Can you work these out from the model? Positions are in its coordinate system, mm. A direction names the side the tool comes from. Round coordinates to 2 decimals unless told otherwise and drop trailing zeros. Loops run counter-clockwise (first coordinate to the right, second up) from the corner with the lowest first, then second, coordinate; pieces in that order, holes last. Notation, with made-up numbers: (49, 35.25) - (103, 35.25) arc R33 ccw to (103, 70.25) - close; hole circle Ø5 at (75, -37.5). An arc over 180 degrees is marked (long way). Answer as CSV lines item,"result".
```python
from build123d import *

# Parameters (mm, degrees)
F0_W     = 127
F0_H     = 76.2
F1_DEPTH = 12
F2_R     = 5
F3_SIZE  = 2
F4_T     = -1


with BuildPart() as f1:
    # F0 (on Top) → F1 (new body)
    with BuildSketch(Plane.XY):
        with Locations((-63.5, -38.1)):
            Rectangle(F0_W, F0_H)
    extrude(amount=F1_DEPTH)

    # F2
    f2_edges = [f1.edges().sort_by_distance(p)[0] for p in [
        (-63.5, -76.2, 0),
    ]]
    fillet(f2_edges, radius=F2_R)

    # F3
    f3_edges = [f1.edges().sort_by_distance(p)[0] for p in [
        (0, -76.2, 8.5),
        (-127, -76.2, 8.5),
    ]]
    chamfer(f3_edges, length=F3_SIZE)

    # F4
    f4_openings = [f1.faces().sort_by_distance(p)[0] for p in [
        (-63.5, -38.084521, 12),
        (-63.5, 0, 6.014035),
    ]]
    offset(amount=F4_T, openings=f4_openings)


solid = f1.part
```
Q1. I'm going to push flat-ended pins straight in: pin 1 Ø4 at (x, z) = (-30.5, 9.5) entering from +Y; pin 2 Ø6 at (x, z) = (-30.5, 6.5) entering from +Y; pin 3 Ø1 at (x, z) = (-82.5, 2) entering from -Y. Where does each tip first touch, or does it pass through?
Checks:
pin 1,"y = -75.2"
pin 2,"y = -74.91"
pin 3,"y = -75.53"
Q2. Imagine slicing it at B-B (x = -43.5). Write out the boundary of the cut face in (y, z), then the cut area to 3 significant figures.
Checks:
outline,"(-76.2, 5) arc R5 ccw to (-71.2, 0) - (0, 0) - (0, 1) - (-71.2, 1) arc R4 cw to (-75.2, 5) - (-75.2, 12) - (-76.2, 12) - close"
area,"85.3 mm²"
Q3. We'd pull the mould along X, two halves only. Please class faces 1 (the conical face through (-126.21, -73.85, 2.29)), 2 (the flat face through (-64, -75.2, 8)), 3 (the flat face through (-63.8, 0, 0.6)): pulls with the +X half, pulls with the -X half, needs draft (parallel to the pull), parting line crosses it, or undercut.
Checks:
face 1,"pulls with the -X half"
face 2,"undercut"
face 3,"needs draft"
Q4. On a 3-axis mill with a long thin cutter (end or side, diameter ignored), from which of +Z, -Z, +X, -X, +Y, -Y can I reach the whole of each face in a straight line? I mean faces 4 (the cylindrical face through (-62.645, -74.059, 2.203)), 5 (the conical face through (-0.76, -73.83, 2.31)). Say none if no direction works.
Checks:
face 4,"+Z, +Y"
face 5,"-Z, +X, -Y"
Q5. If I drill on line 1 along X through (y, z) = (-19.5, 6); line 2 along Z through (x, y) = (-71, -21); line 3 along Y through (x, z) = (-115, 11), over which ranges is the centre line in solid material (lowest first)? Write a range as [from, to].
Checks:
line 1,"[-127, -126], [-1, 0]"
line 2,"[0, 1]"
line 3,"[-76.2, -75.2]"
Q6. Imagine slicing it at C-C (z = 10.25). Write out the boundary of the cut face in (x, y).
Checks:
outline,"(-127, -74.2) - (-125, -76.2) - (-2, -76.2) - (0, -74.2) - (0, 0) - (-1, 0) - (-1, -73.79) - (-2.41, -75.2) - (-124.59, -75.2) - (-126, -73.79) - (-126, 0) - (-127, 0) - close"
Q7. Imagine slicing it at A-A (y = -20.5). Write out the boundary of the cut face in (x, z).
Checks:
outline,"(-127, 2) - (-125, 0) - (-2, 0) - (0, 2) - (0, 12) - (-1, 12) - (-1, 2.41) - (-2.41, 1) - (-124.59, 1) - (-126, 2.41) - (-126, 12) - (-127, 12) - close"
